Input: part model. Units: mm. Frame: model coordinates. Face numbers are marked on the shaded views. A direction names the side the tool comes from. Coordinates: 2 decimals unless noted, no trailing zeros. Write each loop counter-clockwise with the first axis right and the second up, starting at its lowest first coordinate (ties: lowest second). Pieces come first, ordered by that corner, then holes.
1) Pin query (flat end, axial travel): pin 1 Ø8 at (x, y) = (19, 29) entering from +Z; pin 2 Ø4 at (x, y) = (70, 15.5) entering from +Z. Return the tip coordinate at first contact, or that it passes through.
2) Line query: L1, parallel to X at y = 28, z = 23; L2, parallel to Y at x = 1.5, z = 1; L3, parallel to Y at x = 47, z = 18.5. Output: solid intervals per line, ascending.
3) Section query A-A (z = 18). Output: boundary loops of the cut face in (x, y), then the cut area to 3 significant figures.
4) Section query C-C (x = 69.5). Output: boundary loops of the cut face in (y, z), then the cut area to 3 significant figures.
5) Set-up query: the marked faces 4 and 5. Return all of +Z, -Z, +X, -X, +Y, -Y with unobstructed straight access to the full face (end or side cutting, diameter ignored); none if empty.
6) Draft query along X for the marked faces 1, 2 and 3. Return one class per face: pulls with the +X half, pulls with the -X half, needs draft (parallel to the pull), parting line crosses it, or undercut.
7) Section query B-B (y = 12.5). Output: boundary loops of the cut face in (x, z).
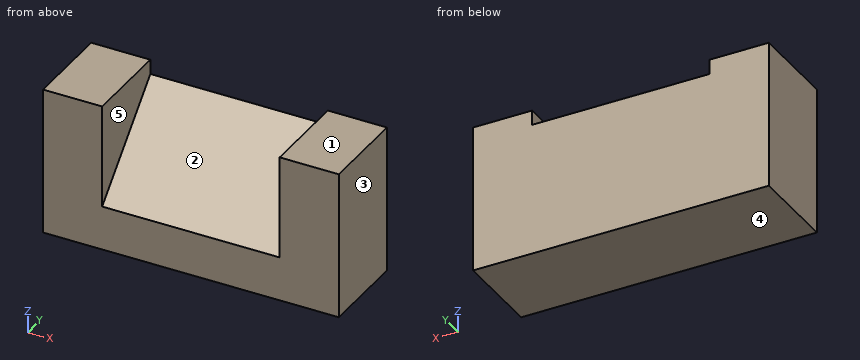
from build123d import *

# Parameters (mm, degrees)
F0_W     = 38.1
F0_H     = 63.5
F1_DEPTH = 76.2
F3_DEPTH = 76.2
F4_W     = 38.1
F4_H     = 63.5
F5_DEPTH = 25.4
F6_W     = 38.1
F6_H     = 63.5
F7_DEPTH = 25.4


with BuildPart() as f1:
    # F0 (on Right) → F1 (new body)
    with BuildSketch(Plane.YZ):
        with Locations((18.2618855059, 0.314003706)):
            Rectangle(F0_W, F0_H)
    extrude(amount=F1_DEPTH)

    # F2 (on face) → F3 (cut)
    with BuildSketch(Plane.YZ.offset(76.2)):
        Polygon((-0.7881144941, 32.064003706), (-0.7881144941, -12.385996294), (37.3118855059, 25.714003706), (37.3118855059, 32.064003706), align=None)
    extrude(amount=-F3_DEPTH, mode=Mode.SUBTRACT)

    # F4 (on face) → F5 (join)
    with BuildSketch(Plane.YZ.offset(76.2)):
        with Locations((18.2618855059, 0.314003706)):
            Rectangle(F4_W, F4_H)
    extrude(amount=F5_DEPTH)

    # F6 (on face) → F7 (join)
    with BuildSketch(Plane(origin=(0, 0, 0), x_dir=(0, -1, 0), z_dir=(-1, 0, 0))):
        with Locations((-18.2618855059, 0.314003706)):
            Rectangle(F6_W, F6_H)
    extrude(amount=F7_DEPTH)


solid = f1.part
Answer:
1. pin 1: stops at z = 21.4
1. pin 2: stops at z = 5.9
2. L1: x = -25.4 to 0, 76.2 to 101.6
2. L2: y = 12.6 to 37.31
2. L3: y = 30.1 to 37.31
3. outline: (-25.4, -0.79) - (0, -0.79) - (0, 29.6) - (76.2, 29.6) - (76.2, -0.79) - (101.6, -0.79) - (101.6, 37.31) - (-25.4, 37.31) - close
3. area: 2,520 mm2
4. outline: (-0.79, -31.44) - (37.31, -31.44) - (37.31, 25.71) - (-0.79, -12.39) - close
4. area: 1,450 mm2
5. face 4: -Z, +X, -X, +Y, -Y
5. face 5: +Z, -Y
6. face 1: needs draft
6. face 2: undercut
6. face 3: pulls with the +X half
7. outline: (-25.4, -31.44) - (101.6, -31.44) - (101.6, 32.06) - (76.2, 32.06) - (76.2, 0.9) - (0, 0.9) - (0, 32.06) - (-25.4, 32.06) - close
